```python
from build123d import *

# Parameters (mm, degrees)
F1_DEPTH = 6.35
F3_DEPTH = 3.175


with BuildPart() as f1:
    # F0 (on Front) → F1 (new body)
    with BuildSketch(Plane.XZ):
        Polygon((-85.428059, -25.659776), (-98.128059, -19.309776), (-98.128059, -44.709776), (-85.428059, -38.359776), (-85.428059, -44.709776), (92.371941, -44.709776), (92.371941, -38.359776), (105.071941, -44.709776), (105.071941, -19.309776), (92.371941, -25.659776), (92.371941, -19.309776), (-85.428059, -19.309776), align=None)
    extrude(amount=F1_DEPTH)

    # F2 (on face) → F3 (cut)
    with BuildSketch(Plane.XZ.offset(6.35)):
        Polygon((16.171941, -19.309776), (-9.228059, -19.309776), (-9.228059, -32.009776), (-9.228059, -44.709776), (16.171941, -44.709776), (16.171941, -32.009776), align=None)
    extrude(amount=-F3_DEPTH, mode=Mode.SUBTRACT)


solid = f1.part
```
Build history of the part. All positions in model axes, mm. A direction names the side the tool comes from. Round coordinates to 2 decimals unless told otherwise and drop trailing zeros. Order: outer loops, then holes, each group sorted by start corner. A loop starts at its lowest first (then second) coordinate and runs counter-clockwise, first axis right, second up. Notation, with made-up numbers: (0, 23) - (16, 23) arc R15 cw to (16, 39) - close; hole circle Ø3 at (43.25, 0.5). An arc over 180 degrees is marked (long way). Use a Markdown table: item, result.
1) Pull direction X, two halves, no side cores. Call faces 1 (the face through (5, -3, -19.31)), 2 (the face through (-91.69, -3.13, -22.53)), 3 (the face through (-98.128, -3, -32)), 4 (the face through (16.172, -5, -32)): pulls with the +X half, pulls with the -X half, needs draft (parallel to the pull), parting line crosses it, or undercut.
Recorded:
| item | result |
|---|---|
| face 1 | needs draft |
| face 2 | undercut |
| face 3 | pulls with the -X half |
| face 4 | undercut |
2) Saw through at A-A on y = -4.25. Write the cut outline in (x, z).
Recorded:
| item | result |
|---|---|
| outline | (-98.13, -44.71) - (-85.43, -38.36) - (-85.43, -44.71) - (-9.23, -44.71) - (-9.23, -19.31) - (-85.43, -19.31) - (-85.43, -25.66) - (-98.13, -19.31) - close; (16.17, -44.71) - (92.37, -44.71) - (92.37, -38.36) - (105.07, -44.71) - (105.07, -19.31) - (92.37, -25.66) - (92.37, -19.31) - (16.17, -19.31) - close |
3) Saw through at B-B on z = -33. Write the cut outline in (x, y) (3 decimals).
Recorded:
| item | result |
|---|---|
| outline | (-98.128, -6.35) - (-9.228, -6.35) - (-9.228, -3.175) - (16.172, -3.175) - (16.172, -6.35) - (105.072, -6.35) - (105.072, 0) - (-98.128, 0) - close |
4) Wall check: L1, parallel to X at y = -5.75, z = -29.25; L2, parallel to Y at x = 6, z = -40 (3 decimals); L3, parallel to X at y = -1.75, z = -41. Give the ranges that are in metal, low to high.
Recorded:
| item | result |
|---|---|
| L1 | x = -98.13 to -9.23, 16.17 to 105.07 |
| L2 | y = -3.175 to 0 |
| L3 | x = -98.13 to -90.71, -85.43 to 92.37, 97.65 to 105.07 |
5) Saw through at D-D on x = 7.5. Write the cut outline in (y, z) (3 decimals).
Recorded:
| item | result |
|---|---|
| outline | (-3.175, -44.71) - (0, -44.71) - (0, -19.31) - (-3.175, -19.31) - close |
6) Saw through at C-C on z = -42.5. Give the number of separate pieces and of enclosed holes in the cut face, and give its area (3 significant figures).
Recorded:
| item | result |
|---|---|
| separate pieces | 3 |
| enclosed holes | 0 |
| area | 1,100 mm² |
7) Tool access for faces 5 (the face through (98.81, -3.13, -22.44)), 6 (the face through (2, 0, -32)), 7 (the face through (-85.428, -3, -41)), 8 (the face through (-9.228, -5, -32)): list every direction of +Z, -Z, +X, -X, +Y, -Y with a clear straight run to the whole face (end or side of a thin tool).
Recorded:
| item | result |
|---|---|
| face 5 | +Z, +Y, -Y |
| face 6 | +Z, -Z, +X, -X, +Y |
| face 7 | -Z, +Y, -Y |
| face 8 | +Z, -Z, -Y |
